```python
from build123d import *

# Parameters (mm, degrees)
SKETCH1_R           = 1
BOSS_EXTRUDE1_DEPTH = 2
BOSS_EXTRUDE2_START = 15.9
BOSS_EXTRUDE2_DEPTH = 15.9
SKETCH3_W           = 12
SKETCH3_H           = 4
BOSS_EXTRUDE3_DEPTH = 10
SKETCH5_R           = 3
BOSS_EXTRUDE4_DEPTH = 3


with BuildPart() as part:
    # Sketch1 → Boss-Extrude1 (new, symmetric)
    with BuildSketch(Plane(origin=(0, 0, 0), x_dir=(1, 0, 0), z_dir=(0, 1, 0))):
        with BuildLine():
            Line((14, 0), (14, 5.9))
            Line((14, 5.9), (36.5, 5.9))
            Line((36.5, 5.9), (36.5, 0))
            Line((36.5, 0), (36.5, -4.438518159))
            Line((36.5, -4.438518159), (41.213519663, -4.438518159))
            Line((41.213519663, -4.438518159), (41.213519663, -3.536214297))
            ThreePointArc((41.213519663, -3.536214297), (41.613535265, -2.452170394), (42.621822841, -1.887794784))
            ThreePointArc((42.621822841, -1.887794784), (59.657919167, -0.157445784), (76.780825793, -0.327016892))
            ThreePointArc((76.780825793, -0.327016892), (79.667666349, -1.303478154), (79.013446705, 1.672983108))
            ThreePointArc((79.013446705, 1.672983108), (44.912555428, 8.893863941), (10.071688353, 9.954942307))
            ThreePointArc((10.071688353, 9.954942307), (5.913323938, 11.457100516), (1.620293164, 12.514626243))
            ThreePointArc((1.620293164, 12.514626243), (0.158700912, 11.813412309), (0.399525234, 10.21030391))
            Line((0.399525234, 10.21030391), (3.821916897, 6.787912247))
            ThreePointArc((3.821916897, 6.787912247), (5.672488258, 3.21348854), (6.62634024, -0.696918803))
            Line((6.62634024, -0.696918803), (6.62634024, -2.438518159))
            ThreePointArc((6.62634024, -2.438518159), (7.212126678, -3.852731721), (8.62634024, -4.438518159))
            Line((8.62634024, -4.438518159), (14, -4.438518159))
            Line((14, -4.438518159), (14, 0))
        make_face()
        with Locations(Location((11.8, 0, 0), (0, 0, 270))):
            Circle(SKETCH1_R, mode=Mode.SUBTRACT)
        with Locations(Location((38.7, 0, 0), (0, 0, 270))):
            Circle(SKETCH1_R, mode=Mode.SUBTRACT)
        with BuildLine():
            Line((43.924254337, 5.25), (43.924254337, 0.65))
            ThreePointArc((43.924254337, 0.65), (56.919306874, 2.126797691), (69.981420933, 1.468391921))
            ThreePointArc((69.981420933, 1.468391921), (57.21989374, 5.199345781), (43.924254337, 5.25))
        make_face(mode=Mode.SUBTRACT)
    extrude(amount=BOSS_EXTRUDE1_DEPTH, both=True)

    # Sketch2 → Boss-Extrude2 (add)
    with BuildSketch(Plane(origin=(0, 2, 0), x_dir=(1, 0, 0), z_dir=(0, 1, 0)).offset(BOSS_EXTRUDE2_START)):
        with BuildLine():
            Line((14, 5.9), (14, 10.146104419))
            ThreePointArc((14, 10.146104419), (19.999270016, 10.285681215), (26, 10.241385974))
            Line((26, 10.241385974), (26, 5.9))
            Line((26, 5.9), (14, 5.9))
        make_face()
    extrude(amount=-BOSS_EXTRUDE2_DEPTH)

    # Sketch3 → Boss-Extrude3 (add)
    with BuildSketch(Plane.XY.offset(-5.9)):
        with Locations((20, 15.9)):
            Rectangle(SKETCH3_W, SKETCH3_H)
    extrude(amount=BOSS_EXTRUDE3_DEPTH)

    # Sketch5 → Boss-Extrude4 (add)
    with BuildSketch(Plane(origin=(0, 17.9, 0), x_dir=(1, 0, 0), z_dir=(0, 1, 0))):
        with Locations(Location((19.9, 0, 0), (0, 0, 270))):
            Circle(SKETCH5_R)
    extrude(amount=BOSS_EXTRUDE4_DEPTH)


solid = part.part
```
Can you work these out from the model? Positions are in its coordinate system, mm. A direction names the side the tool comes from. Round coordinates to 2 decimals unless told otherwise and drop trailing zeros. Order: outer loops, then holes, each group sorted by start corner. A loop starts at its lowest first (then second) coordinate and runs counter-clockwise, first axis right, second up. Notation, with made-up numbers: (85, -37) -> (134, -37) arc R33 ccw to (134, 0) -> close; hole circle Ø2 at (52, -19.5). An arc over 180 degrees is marked (long way). Return JSON: item names as keys, results as strings. Group by question number.
1. If we section it at A-A, the plane x = 62: Write out the boundary of the cut face in (y, z).
2. If we section it at C-C, the plane y = 4.5: Write out the boundary of the cut face in (x, z).
3. If we section it at B-B, the plane x = 19.9: Write out the boundary of the cut face in (y, z).
4. Will these pins go through, and if not, where does the flat tip stop? pin 1 (3 mm diameter, centred on x = 15, y = 1.5, fed in from -Z); pin 2 (3 mm diameter, centred on y = 11.5, z = -8.5, fed in from +X); pin 3 (4.5 mm diameter, centred on y = 0.5, z = -3, fed in from -X); pin 4 (1 mm diameter, centred on x = 45.5, z = -2, fed in from -Y).
5. I need wall thicknesses on line 1 (Y direction, x = 39, z = 2); line 2 (Y direction, x = 22.5, z = -3); line 3 (Z direction, x = 22.5, y = 17.5). Which ranges of each line are inside material? Lowest first, please. Write a range as [from, to].
6. Which directions (+Z, -Z, +X, -X, +Y, -Y) give clear straight access to the entire face, cutting with the end or side of a thin tool? Please do faces 4 (the face through (8, 2, -4)), 5 (the face through (6.626, 0, 2)), 6 (the face through (23, 4, -5.9)), 7 (the face through (20, 20.9, 0)), 8 (the face through (26, 11.6, -6.4)).
7. We'd pull the mould along X, two halves only. Please class faces 1 (the face through (16.97, 19.38, -0.65)), 2 (the face through (39, 0, 4.439)), 3 (the face through (79.629, 0.028, 1.337)): released by +X, released by -X, zero draft, split by the parting line, or undercut.
Output values:
{
 "1": {"outline": "(-2, -6.07) -> (2, -6.07) -> (2, -4.25) -> (-2, -4.25) -> close; (-2, -2.13) -> (2, -2.13) -> (2, 0.07) -> (-2, 0.07) -> close"},
 "2": {"outline": "(14, -10.15) arc R195.84 ccw to (26, -10.24) -> (26, -5.9) -> (14, -5.9) -> close"},
 "3": {"outline": "(-2, -10.28) -> (17.9, -10.28) -> (17.9, -3) -> (20.9, -3) -> (20.9, 3) -> (17.9, 3) -> (17.9, 4.1) -> (13.9, 4.1) -> (13.9, -5.9) -> (-2, -5.9) -> close"},
 "4": {"pin 1": "z = -10.23", "pin 2": "x = 26", "pin 3": "x = 4.75", "pin 4": "through"},
 "5": {"line 1": "[-2, 2]", "line 2": "[13.9, 17.9]", "line 3": "[-10.29, 4.1]"},
 "6": {"face 4": "+Z, -Z, -X, +Y", "face 5": "+Z, -X, +Y, -Y", "face 6": "+Z, -Y", "face 7": "+Z, -Z, +X, -X, +Y", "face 8": "+Z, -Z, +X, +Y"},
 "7": {"face 1": "split by the parting line", "face 2": "zero draft", "face 3": "undercut"}
}
